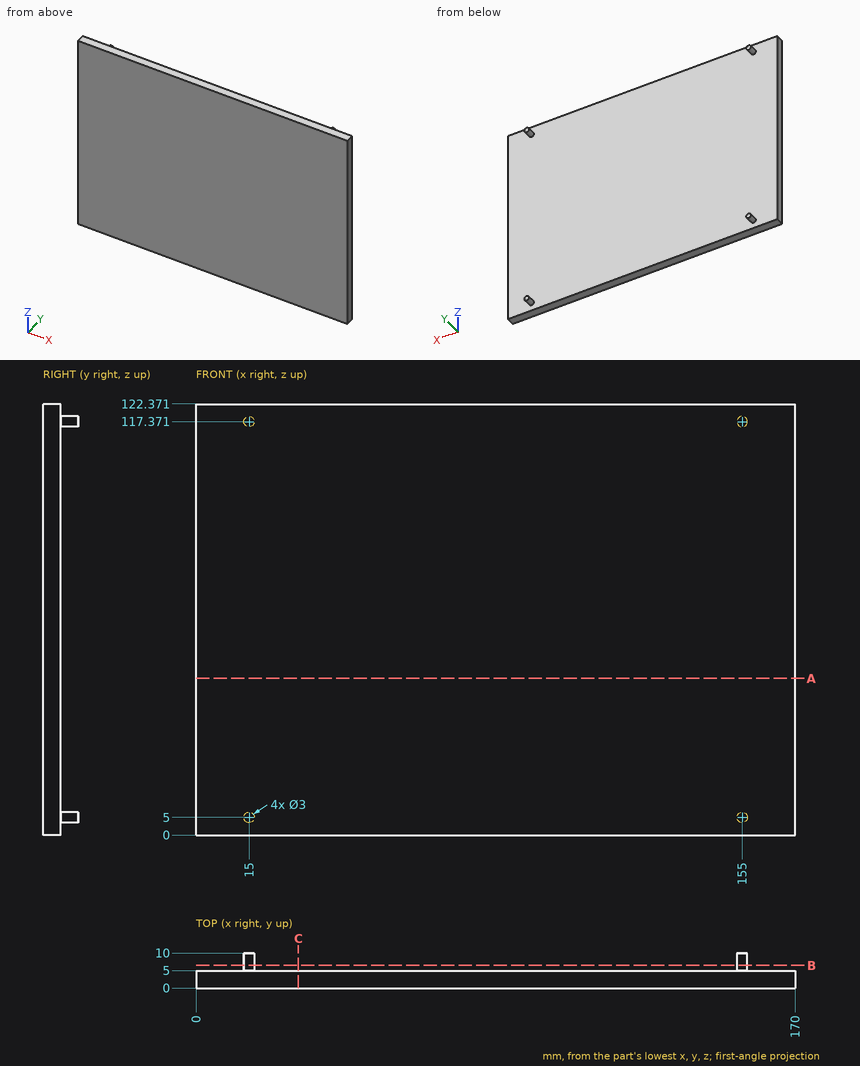
The figure shows three views and two pictorial views of one solid part (mm, origin at its lowest corner). Answer the questions. Round coordinates to 2 decimals unless told otherwise and drop trailing zeros. Order: outer loops, then holes, each group sorted by start corner. A loop starts at its lowest first (then second) coordinate and runs counter-clockwise, first axis right, second up. Notation, with made-up numbers: (54.5, 19) - (104.5, 19) arc R30 ccw to (104.5, 42) - close; hole circle Ø3 at (-37.5, 3.5). An arc over 180 degrees is marked (long way). Write item = value, one per line. Start each with the question number.
1) Section B-B, the plane y = 6.5 is taken. Write down the section's boundary in (x, z).
2) Straight lines are drawn through the part: L1, parallel to Y at x = 14, z = 48.5; L2, parallel to Z at x = 156, y = 8.75. For each, find the intervals that lie inside material, in ascending order.
3) Section C-C, the plane x = 29 is taken. Write down the section's boundary in (y, z).
4) Section A-A, the plane z = 44.5 is taken. Write down the section's boundary in (x, y), plus the area to 3 significant figures.
Results list:
q1.outline = circle Ø3 at (15, 5); circle Ø3 at (15, 117.37); circle Ø3 at (155, 5); circle Ø3 at (155, 117.37)
q2.L1 = 0 to 5
q2.L2 = 3.88 to 6.12, 116.25 to 118.49
q3.outline = (0, 0) - (5, 0) - (5, 122.37) - (0, 122.37) - close
q4.outline = (0, 0) - (170, 0) - (170, 5) - (0, 5) - close
q4.area = 850 mm^2
